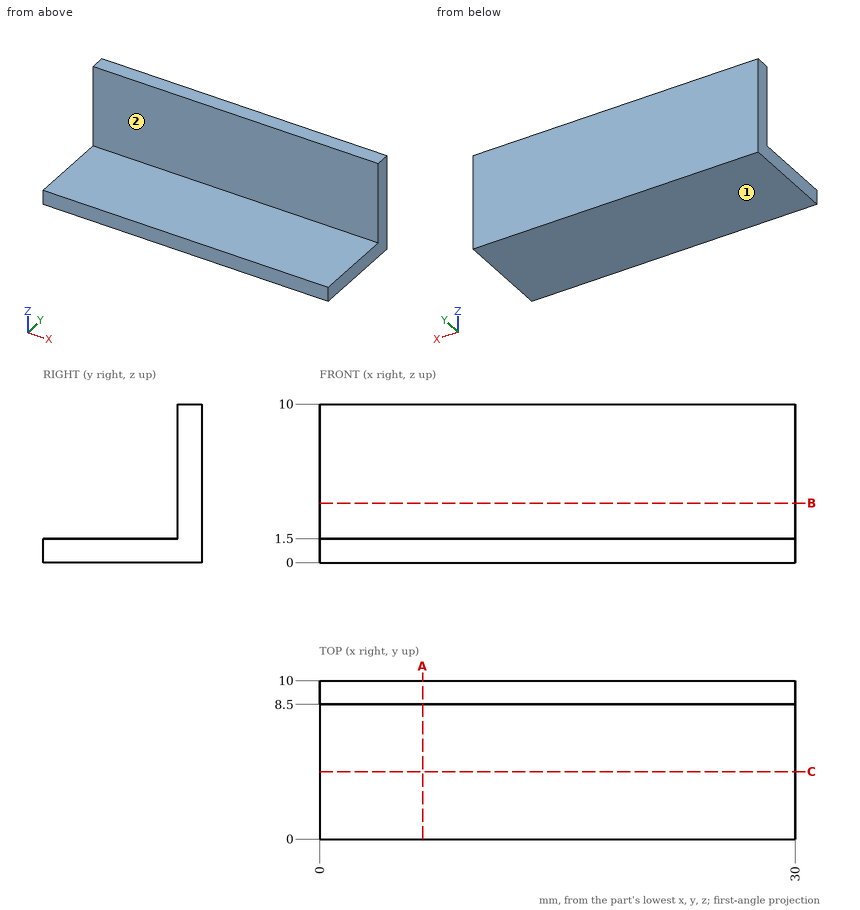
Check sheet for the drawn part. Datum: minimum x, y, z corner. Units: mm. A direction names the side the tool comes from. Round coordinates to 2 decimals unless told otherwise and drop trailing zeros. Order: outer loops, then holes, each group sorted by start corner. A loop starts at its lowest first (then second) coordinate and runs counter-clockwise, first axis right, second up. Notation, with made-up numbers: M -16,-34 L -1,-34 A15 cw -1,-20 Z; hole C -35.75,79 d1. An arc over 180 degrees is marked long. Write each question's results on one line, items separated by ' | '. Start each with the question number.
1. Cross-section at C-C on y = 4.25. Record the boundary of the cut face in (x, z).
2. Go/stop test with flat-tipped pins: P1, Ø4, axis at x = 11, y = 6, coming from the +Z side; P2, Ø6, axis at x = 14, z = 5, coming from the -Y side. Record where each tip stops, or that it passes through.
3. Cross-section at B-B on z = 3.75. Record the boundary of the cut face in (x, y), plus the area to 3 significant figures.
4. Material ranges on L1, parallel to Z at x = 25.75, y = 6; L2, parallel to Y at x = 7.25, z = 8, recorded low to high. Write a range as from..to.
5. Set-up check for the marked faces 1 and 2: record each of +Z, -Z, +X, -X, +Y, -Y from which the full face is reachable in a straight line by a thin tool's end or side.
6. Cross-section at A-A on x = 6.5. Record the boundary of the cut face in (y, z).
Resolved:
1) outline: M 0,0 L 30,0 L 30,1.5 L 0,1.5 Z
2) P1: z = 1.5 | P2: y = 8.5
3) outline: M 0,8.5 L 30,8.5 L 30,10 L 0,10 Z | area: 45.0 mm2
4) L1: 0..1.5 | L2: 8.5..10
5) face 1: -Z, +X, -X, +Y, -Y | face 2: +Z, +X, -X, -Y
6) outline: M 0,0 L 10,0 L 10,10 L 8.5,10 L 8.5,1.5 L 0,1.5 Z
